For this review, take the finished solid that the model builds, in its own axes (mm). Coordinates: 2 decimals unless noted, no trailing zeros. Loops run counter-clockwise (first coordinate to the right, second up) from the corner with the lowest first, then second, coordinate; pieces in that order, holes last. Notation, with made-up numbers: (-28, 29) -> (-15, 29) arc R28 cw to (-15, 53) -> close; hole circle Ø10 at (32, 43.5). An arc over 180 degrees is marked (long way). One line per item, written item: value.
from build123d import *
from build123d.topology import SkipClean

# Parameters (mm, degrees)
BOSS_EXTRUDE1_DEPTH      = 3
BOSS_EXTRUDE1_DEPTH_BACK = 1.5
SKETCH1_R                = 8
SKETCH2_W                = 16
SKETCH2_H                = 50
BOSS_EXTRUDE2_DEPTH      = 1.5
CUT_EXTRUDE1_REACH       = 52.836
SKETCH3_R                = 1.5
CUT_EXTRUDE3_REACH       = 52.725
SKETCH5_R                = 1.5


with BuildPart() as part:
    # Sketch1 → Boss-Extrude1 (new, two sides: drawn at the far end of the back side and taken through both)
    with BuildSketch(Plane(origin=(0, 0, 0), x_dir=(1, 0, 0), z_dir=(0, 1, 0)).offset(-BOSS_EXTRUDE1_DEPTH_BACK)):
        with Locations(Location((0, 0, 0), (0, 0, 270))):
            Circle(SKETCH1_R)
    extrude(amount=BOSS_EXTRUDE1_DEPTH + BOSS_EXTRUDE1_DEPTH_BACK)

    # Sketch2 → Boss-Extrude2 (add, symmetric)
    with BuildSketch(Plane(origin=(0, 0, 0), x_dir=(1, 0, 0), z_dir=(0, 1, 0))):
        with Locations((0, -25)):
            Rectangle(SKETCH2_W, SKETCH2_H)
    extrude(amount=BOSS_EXTRUDE2_DEPTH, both=True)

    # Sketch3 → Cut-Extrude1 (cut, up to next)
    with BuildSketch(Plane(origin=(0, -1.5, 0), x_dir=(-1, 0, 0), z_dir=(0, -1, 0)), mode=Mode.PRIVATE) as cut_extrude1_sk1:
        with Locations(Location((2.503073418, -45.5, 0), (0, 0, 90))):
            Circle(SKETCH3_R)
    cut_extrude1_tool1 = extrude(cut_extrude1_sk1.sketch, amount=-CUT_EXTRUDE1_REACH, mode=Mode.PRIVATE) & part.part
    # Sketch3 → Cut-Extrude1 (cut, up to next)
    with BuildSketch(Plane(origin=(0, -1.5, 0), x_dir=(-1, 0, 0), z_dir=(0, -1, 0)), mode=Mode.PRIVATE) as cut_extrude1_sk2:
        with Locations(Location((-2.503073418, -45.5, 0), (0, 0, 90))):
            Circle(SKETCH3_R)
    cut_extrude1_tool2 = extrude(cut_extrude1_sk2.sketch, amount=-CUT_EXTRUDE1_REACH, mode=Mode.PRIVATE) & part.part
    add(cut_extrude1_tool1.solids().sort_by_distance((-2.503073, -1.5, 45.5))[0], mode=Mode.SUBTRACT)
    add(cut_extrude1_tool2.solids().sort_by_distance((2.503073, -1.5, 45.5))[0], mode=Mode.SUBTRACT)

    # Sketch4 → Cut-Revolve21 (revolve, cut)
    with SkipClean():  # the faces are left unmerged after this step: merging them gives an invalid solid
        with BuildSketch(Plane(origin=(0, -1.5, 0), x_dir=(-1, 0, 0), z_dir=(0, -1, 0))):
            with BuildLine():
                ThreePointArc((3.3, 0), (0, 3.3), (-3.3, 0))
                Line((-3.3, 0), (3.3, 0))
            make_face()
            with BuildLine():
                Line((3.3, 0), (-3.3, 0))
                ThreePointArc((-3.3, 0), (0, -3.3), (3.3, 0))
            make_face()
        revolve(axis=Axis((3.3, -1.5, 0), (-1, 0, 0)), mode=Mode.SUBTRACT)
    add(part.part.scale(1), mode=Mode.REPLACE)  # the faces are merged on a copy

    # Sketch5 → Cut-Extrude3 (cut, up to next)
    with BuildSketch(Plane(origin=(0, 1.5, 0), x_dir=(1, 0, 0), z_dir=(0, 1, 0)), mode=Mode.PRIVATE) as cut_extrude3_sk1:
        with Locations(Location((0, -25, 0), (0, 0, 270))):
            Circle(SKETCH5_R)
    cut_extrude3_tool1 = extrude(cut_extrude3_sk1.sketch, amount=-CUT_EXTRUDE3_REACH, mode=Mode.PRIVATE) & part.part
    add(cut_extrude3_tool1.solids().sort_by_distance((0, 1.5, 25))[0], mode=Mode.SUBTRACT)


solid = part.part
1. Insertion check: pin 1 Ø1.8 at (x, z) = (2.5, 45.5) entering from -Y; pin 2 Ø2 at (x, z) = (-6.5, 13.5) entering from +Y. Each pin has a flat end and moves straight along its axis. Give the tip position at first contact, or say it passes through.
Return value:
pin 1: passes through
pin 2: stops at y = 1.5
2. The part is to be moulded in two halves that separate along X. For faces 1 (the flat face through (0, 1.5, 30)), 2 (the cylindrical face through (0, 1, -8)), 3 (the cylindrical face through (-2.44, -0.02, 47)), 4 (the cylindrical face through (2.57, -0.02, 47)), say which applies: pulls with the +X half, pulls with the -X half, needs draft (parallel to the pull), parting line crosses it, or undercut.
Return value:
face 1: needs draft
face 2: parting line crosses it
face 3: undercut
face 4: undercut
3. Take a section at D-D, the plane y = -0.7. Give the boundary of the cut face in (x, z).
Return value:
outline: (-8, 0) arc R8 ccw to (8, 0) -> (8, 50) -> (-8, 50) -> close; hole circle Ø3 at (-2.5, 45.5); hole circle Ø6.4 at (0, 0); hole circle Ø3 at (0, 25); hole circle Ø3 at (2.5, 45.5)
4. Take a section at A-A, the plane x = 0. Give the boundary of the cut face in (y, z).
Return value:
outline: (-1.5, -8) -> (3, -8) -> (3, 8) -> (1.5, 8) -> (1.5, 23.5) -> (-1.5, 23.5) -> (-1.5, 3.3) arc R3.3 cw to (-1.5, -3.3) -> close; (-1.5, 26.5) -> (1.5, 26.5) -> (1.5, 50) -> (-1.5, 50) -> close
5. To check wall thickness, follow probe 1 along X at (y, z) = (-0.6, 45.5); probe 2 along X at (y, z) = (0.4, 25); probe 3 along Y at (x, z) = (-4.25, 45). State the ranges of each line that lie inside material, in increasing order. Write a range as from..to.
Return value:
probe 1: x = -8..-4, -1..1, 4..8
probe 2: x = -8..-1.5, 1.5..8
probe 3: y = -1.5..1.5
6. Take a section at C-C, the plane z = 25. Give the boundary of the cut face in (x, y).
Return value:
outline: (-8, -1.5) -> (-1.5, -1.5) -> (-1.5, 1.5) -> (-8, 1.5) -> close; (1.5, -1.5) -> (8, -1.5) -> (8, 1.5) -> (1.5, 1.5) -> close
7. Take a section at B-B, the plane z = 45.5. Give the boundary of the cut face in (x, y).
Return value:
outline: (-8, -1.5) -> (-4, -1.5) -> (-4, 1.5) -> (-8, 1.5) -> close; (-1, -1.5) -> (1, -1.5) -> (1, 1.5) -> (-1, 1.5) -> close; (4, -1.5) -> (8, -1.5) -> (8, 1.5) -> (4, 1.5) -> close
